Autodesk Inventor part; units mm, degrees
ref_plane "YZ Plane" through (0, 0, 0) normal (1, 0, 0) x (0, 1, 0)
ref_plane "XZ Plane" through (0, 0, 0) normal (0, 1, 0) x (-1, 0, 0)
ref_plane "XY Plane" through (0, 0, 0) normal (0, 0, 1) x (1, 0, 0)
sketch "Sketch1" plane through (0, 0, 0) normal (0, 0, 1) x (1, 0, 0)
  line L0 (-40, -40) -> (40, -40)
  line L1 (40, -40) -> (40, 40)
  line L2 (40, 40) -> (-40, 40)
  line L3 (-40, 40) -> (-40, -40)
  line L4 (-40, -40) -> (40, 40) construction
  line L5 (40, -40) -> (-40, 40) construction
  point P0 (0, 0)
  dimension "d0" = 80
  dimension "d1" = 80
extrude "Extrusion1" add sketch "Sketch1" along normal blind 6
sketch "Sketch2" plane through (0, 0, 6) normal (0, 0, 1) x (1, 0, 0)
  arc A0 (-37, 21.1) -> (-40, 18.1) centre (-37, 18.1) ccw
  line L0 (-40, 14.1) -> (-40, 18.1)
  arc A1 (-40, 14.1) -> (-37, 11.1) centre (-37, 14.1) ccw
  line L1 (-37, 11.1) -> (-31.2426, 11.1)
  arc A2 (-29.1213, 10.2213) -> (-31.2426, 11.1) centre (-31.2426, 8.1) ccw
  line L2 (-29.1213, 10.2213) -> (-20.8787, 1.9787)
  arc A3 (-20, -0.1426) -> (-20.8787, 1.9787) centre (-23, -0.1426) ccw
  line L3 (-20, -0.1426) -> (-20, -37)
  arc A4 (-20, -37) -> (-17, -40) centre (-17, -37) ccw
  line L4 (-17, -40) -> (17, -40)
  arc A5 (17, -40) -> (20, -37) centre (17, -37) ccw
  line L5 (20, -37) -> (20, -0.1426)
  arc A6 (20.8787, 1.9787) -> (20, -0.1426) centre (23, -0.1426) ccw
  line L6 (20.8787, 1.9787) -> (29.1213, 10.2213)
  arc A7 (31.2426, 11.1) -> (29.1213, 10.2213) centre (31.2426, 8.1) ccw
  line L7 (31.2426, 11.1) -> (37, 11.1)
  arc A8 (37, 11.1) -> (40, 14.1) centre (37, 14.1) ccw
  line L8 (40, 14.1) -> (40, 18.1)
  arc A9 (40, 18.1) -> (37, 21.1) centre (37, 18.1) ccw
  line L9 (-37, 21.1) -> (37, 21.1)
  line L10 (10.1, -30) -> (10.1, 11.1)
  line L11 (10.1, -30) -> (-10.1, -30)
  line L12 (-10.1, -30) -> (-10.1, 11.1)
  line L13 (-10.1, 11.1) -> (10.1, 11.1)
  circle A10 centre (15, -35) radius 2
  circle A11 centre (-15, -15) radius 2
  circle A12 centre (-15, -35) radius 2
  circle A13 centre (15, -15) radius 2
  circle A14 centre (-15, 5) radius 2
  circle A15 centre (15, 5) radius 2
  line L14 (-40, -40) -> (40, -40)
  line L15 (40, -40) -> (40, 40)
  line L16 (40, 40) -> (-40, 40)
  line L17 (-40, 40) -> (-40, -40)
  line L18 (-40, -40) -> (40, 40) construction
  line L19 (40, -40) -> (-40, 40) construction
  line L20 (40, 40) -> (-40, 40)
  line L21 (40, -40) -> (40, 40)
  line L22 (-10.1, -30) -> (10.1, -30)
  line L23 (10.1, -30) -> (10.1, 11.1)
  line L24 (10.1, 11.1) -> (-10.1, 11.1)
  line L25 (-10.1, 11.1) -> (-10.1, -30)
  line L26 (-10.1, -30) -> (10.1, 11.1) construction
  line L27 (10.1, -30) -> (-10.1, 11.1) construction
  point P0 (0, 0)
  point P1 (40, 14.1)
  point P2 (0, -9.45)
sketch "Sketch3" plane through (0, 0, 6) normal (0, 0, 1) x (1, 0, 0)
  line L0 (37, 14.1) -> (37, 21.1)
  line L1 (23, 14.1) -> (37, 14.1)
  arc A0 (23, 14.1) -> (17, 8.1) centre (23, 8.1) ccw
  line L2 (17, -37) -> (17, 8.1)
  line L3 (-17, -37) -> (17, -37)
  line L4 (-17, 8.1) -> (-17, -37)
  arc A1 (-17, 8.1) -> (-23, 14.1) centre (-23, 8.1) ccw
  line L5 (-37, 14.1) -> (-23, 14.1)
  line L6 (-37, 21.1) -> (-37, 14.1)
  line L7 (37, 21.1) -> (-37, 21.1)
  circle A2 centre (0, -20) radius 7.5
  circle A3 centre (-7.525, -27.5) radius 2
  circle A4 centre (7.525, -27.5) radius 2
  circle A5 centre (7.525, 7.6) radius 2
  circle A6 centre (-7.525, 7.6) radius 2
  circle A7 centre (7.525, -7.5) radius 2
  circle A8 centre (-7.525, -7.5) radius 2
  circle A9 centre (0, -20) radius 11
  point P0 (0, 0)
  dimension "d4" = 22
extrude "Extrusion2" cut sketch "Sketch2" against normal blind 7 contours A0 L17 L16 L15 A9 L9 | A1 L1 A2 L2 A3 L3 A4 L14 L17 | L15 L14 A5 L5 A6 L6 A7 L7 A8 | A10 | A11 | A12 | A13 | A14 | A15
extrude "Extrusion3" cut sketch "Sketch3" against normal blind 7 contours A2 | A3 A9 | A3 A9 A4 | A4 A9 picked at (-7.1985, -27.22) picked at (7.2207, -27.1967)
sketch "Sketch4" plane through (0, 0, 6) normal (0, 0, 1) x (1, 0, 0)
  circle A0 centre (-15, 5) radius 2
  circle A1 centre (15, 5) radius 2
  circle A2 centre (-15, -15) radius 2
  circle A3 centre (15, -15) radius 2
  circle A4 centre (-15, -35) radius 2
  circle A5 centre (15, -35) radius 2
  circle A6 centre (15, 5) radius 3.5
  circle A7 centre (15, -15) radius 3.5
  circle A8 centre (15, -35) radius 3.5
  circle A9 centre (-15, -35) radius 3.5
  circle A10 centre (-15, -15) radius 3.5
  circle A11 centre (-15, 5) radius 3.5
  point P0 (0, 0)
  dimension "d9" = 7
  dimension "d10" = 7
  dimension "d11" = 7
  dimension "d12" = 7
  dimension "d13" = 7
  dimension "d14" = 7
extrude "Extrusion4" cut sketch "Sketch4" against normal blind 3
properties part number "stopper_motor_bracket_cover"
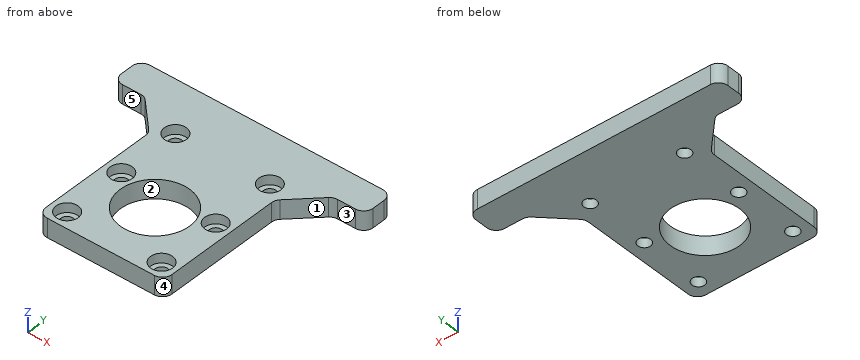
Check sheet for the modelled part. Datum: model origin and axes. Units: mm. Face numbers are marked on the shaded views. A direction names the side the tool comes from. Round coordinates to 2 decimals unless told otherwise and drop trailing zeros. Loops run counter-clockwise (first coordinate to the right, second up) from the corner with the lowest first, then second, coordinate; pieces in that order, holes last. Notation, with made-up numbers: M 42.5,59 L 89.5,59 A21 cw 89.5,76 Z; hole C 74,64 d2. An arc over 180 degrees is marked long. One line per question, with ' | ' between items. Start each with the question number.
Item 1: Gauge pin test, flat ends, axial feed: pin 1 Ø5.5 at (x, y) = (-15, 5) entering from +Z; pin 2 Ø1 at (y, z) = (9, 5) entering from -X; pin 3 Ø20 at (x, y) = (0, -20) entering from +Z. Record the tip position at first contact, or that the pin passes through.
Item 2: Set-up check for the marked faces 4 and 5: record each of +Z, -Z, +X, -X, +Y, -Y from which the full face is reachable in a straight line by a thin tool's end or side.
Item 3: Section check D-D (x = 0). Record the boundary of the cut face in (y, z).
Item 4: Release check for a two-part mould opening along X. For the marked faces 1, 2 and 3 record: released by +X, released by -X, zero draft, split by the parting line, or undercut.
Item 5: Scan lines: probe 1 along Y at (x, z) = (15, 1.6); probe 2 along Y at (x, z) = (15, 5.35); probe 3 along X at (y, z) = (-36.5, 5.55). Record each from-to range of solid material in increasing order.
Item 6: Section check A-A (y = -35). Record the boundary of the cut face in (x, z).
Item 7: Section check B-B (x = -15). Record the boundary of the cut face in (y, z).
Item 8: Section check C-C (z = 1.45). Record the boundary of the cut face in (x, y), and give its area (3 significant figures).
Worked out:
1) pin 1: z = 3 | pin 2: x = -28.4 | pin 3: through
2) face 4: +Z, -Z, +X, -Y | face 5: +Z, -Z, -X, -Y
3) outline: M -40,0 L -31,0 L -31,6 L -40,6 Z; M -9,0 L 21.1,0 L 21.1,6 L -9,6 Z
4) face 1: released by +X | face 2: undercut | face 3: zero draft
5) probe 1: -40 to -37, -33 to -17, -13 to 3, 7 to 21.1 | probe 2: -40 to -38.5, -31.5 to -18.5, -11.5 to 1.5, 8.5 to 21.1 | probe 3: -20 to -18.16, -11.84 to 11.84, 18.16 to 20
6) outline: M -20,0 L -17,0 L -17,3 L -18.5,3 L -18.5,6 L -20,6 Z; M -13,0 L 13,0 L 13,3 L 11.5,3 L 11.5,6 L -11.5,6 L -11.5,3 L -13,3 Z; M 17,0 L 20,0 L 20,6 L 18.5,6 L 18.5,3 L 17,3 Z
7) outline: M -40,0 L -37,0 L -37,3 L -38.5,3 L -38.5,6 L -40,6 Z; M -33,0 L -17,0 L -17,3 L -18.5,3 L -18.5,6 L -31.5,6 L -31.5,3 L -33,3 Z; M -13,0 L 3,0 L 3,3 L 1.5,3 L 1.5,6 L -11.5,6 L -11.5,3 L -13,3 Z; M 7,0 L 21.1,0 L 21.1,6 L 8.5,6 L 8.5,3 L 7,3 Z
8) outline: M -40,14.1 A3 ccw -37,11.1 L -31.24,11.1 A3 cw -29.12,10.22 L -20.88,1.98 A3 cw -20,-0.14 L -20,-37 A3 ccw -17,-40 L 17,-40 A3 ccw 20,-37 L 20,-0.14 A3 cw 20.88,1.98 L 29.12,10.22 A3 cw 31.24,11.1 L 37,11.1 A3 ccw 40,14.1 L 40,18.1 A3 ccw 37,21.1 L -37,21.1 A3 ccw -40,18.1 Z; hole C -15,-35 d4; hole C -15,-15 d4; hole C -15,5 d4; hole C 0,-20 d22; hole C 15,-35 d4; hole C 15,-15 d4; hole C 15,5 d4 | area: 2,480 mm^2
